Could you check a few things on this drawing? It's one solid part, dimensions in mm from its lowest x, y, z. Coordinates: 2 decimals unless noted, no trailing zeros. Write each loop counter-clockwise with the first axis right and the second up, starting at its lowest first coordinate (ties: lowest second). Pieces come first, ordered by that corner, then holes.
Item 1: I want a section at C-C (z = 2.3). Count the separate pieces of the cut face and the enclosed holes in it, and give its area (3 significant figures).
Item 2: Please list where this line runs through material, in increasing order: line 1 (Y direction, x = 61, z = 0.85).
Item 3: I want a section at A-A (x = 150). Please give me the cut outline in (y, z), and give its area (3 significant figures).
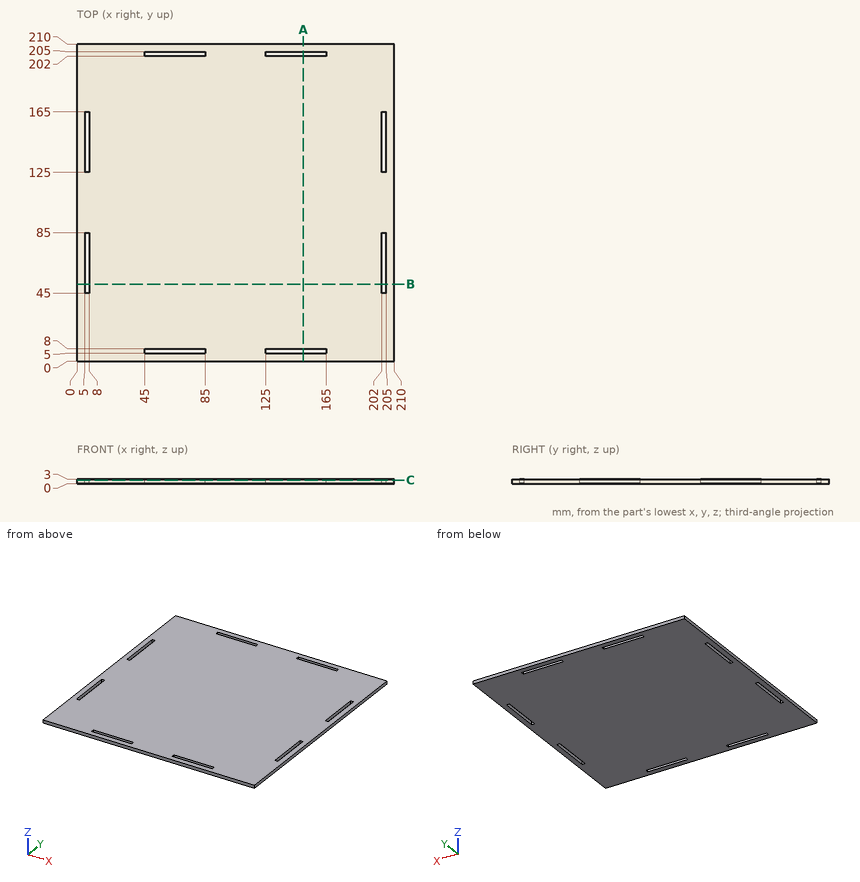
Answer:
1. separate pieces: 1
1. enclosed holes: 8
1. area: 43,100 mm2
2. line 1: y = 0 to 5, 8 to 202, 205 to 210
3. outline: (0, 0) - (5, 0) - (5, 3) - (0, 3) - close; (8, 0) - (202, 0) - (202, 3) - (8, 3) - close; (205, 0) - (210, 0) - (210, 3) - (205, 3) - close
3. area: 612 mm2
